The figure shows three views and two pictorial views of one solid part (mm, origin at its lowest corner). Answer the questions. A direction names the side the tool comes from. Coordinates: 2 decimals unless noted, no trailing zeros. Write each loop counter-clockwise with the first axis right and the second up, starting at its lowest first coordinate (ties: lowest second). Pieces come first, ordered by that corner, then holes.
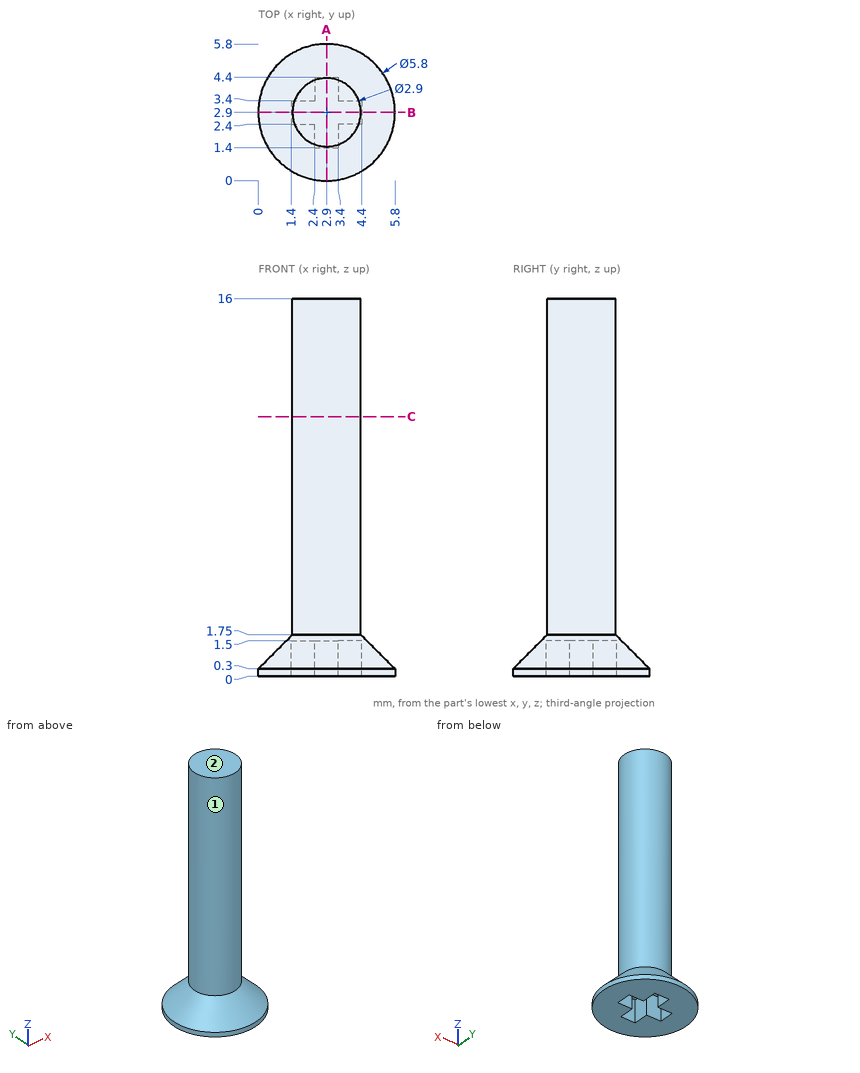
1. Section A-A on x = 2.9 is taken. Give the vertices of the cut face in (y, z), then the cut area to 3 significant figures.
Results found:
outline: (0, 0) - (1.4, 0) - (1.4, 1.5) - (4.4, 1.5) - (4.4, 0) - (5.8, 0) - (5.8, 0.3) - (4.35, 1.75) - (4.35, 16) - (1.45, 16) - (1.45, 1.75) - (0, 0.3) - close
area: 44.9 mm2
2. Section C-C on z = 11 is taken. Give the vertices of the cut face in (x, y), then the cut area to 3 significant figures.
Results found:
outline: circle Ø2.9 at (2.9, 2.9)
area: 6.61 mm2
3. Find the intervals of material crossed by L1, parallel to Y at x = 2.8, z = 2.5; L2, parallel to Z at x = 2.5, y = 1.6; L3, parallel to Z at x = 5, y = 1.1, in increasing order.
Results found:
L1: y = 1.45 to 4.35
L2: z = 1.5 to 16
L3: z = 0 to 0.43
4. Flat-ended cylindrical pins translate along their axes: P1, Ø3, axis at x = 2.5, z = 6.5, coming from the +Y side; P2, Ø0.5, axis at x = 3, z = 1, coming from the -Y side; P3, Ø1.1, axis at y = 4, z = 0.5, coming from the +X side. Find the tip coordinate at first contact, or state that the pin passes through.
Results found:
P1: stops at y = 4.35
P2: stops at y = 0.45
P3: stops at x = 5.74
5. A tool of negligible diameter and unlimited length cuts with its end or side. For the marked faces 1 and 2, from which of +Z, -Z, +X, -X, +Y, -Y can it reach the whole face along a straight path? Write none if from no direction.
Results found:
face 1: +Z
face 2: +Z, +X, -X, +Y, -Y
